```python
from build123d import *

# Parameters (mm, degrees)
BOSS_EXTRUDE1_DEPTH = 5
CUT_EXTRUDE1_DEPTH  = 44.153794735


with BuildPart() as part:
    # Sketch1 → Boss-Extrude1 (new body)
    with BuildSketch(Plane(origin=(0, 0, 0), x_dir=(1, 0, 0), z_dir=(0, 1, 0))):
        Polygon((-41, -5), (-41, 5), (-38, 5), (-38, 7.5), (-28.5, 7.5), (-28.5, 12.5), (-9.5, 12.5), (-9.5, 7.5), (0, 7.5), (0, -7.5), (-38, -7.5), (-38, -5), align=None)
    boss_extrude1 = extrude(amount=BOSS_EXTRUDE1_DEPTH)

    # Mirror1: Boss-Extrude1 across plane
    add(boss_extrude1.mirror(Plane(origin=(0, 5, -7.5), x_dir=(0, 0, 1), z_dir=(-1, 0, 0))))

    # Sketch4 → Cut-Extrude1 (cut, through all)
    with BuildSketch(Plane(origin=(0, 5, 0), x_dir=(1, 0, 0), z_dir=(0, 1, 0))):
        with BuildLine():
            Line((-33, -7.5), (33, -7.5))
            ThreePointArc((33, -7.5), (0, -2.5), (-33, -7.5))
        make_face()
    extrude(amount=-CUT_EXTRUDE1_DEPTH, mode=Mode.SUBTRACT)


solid = part.part
```
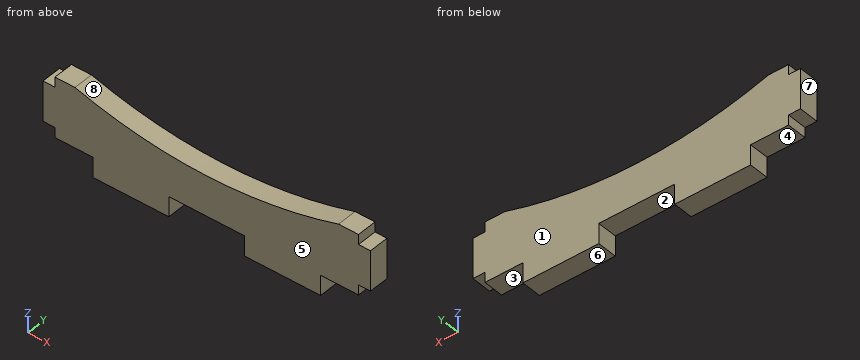
Geometry: final body of the model. Coordinates: model frame, mm. Face numbers are marked on the shaded views. A direction names the side the tool comes from. Give positions to 0.01 mm unless a question says otherwise; leave off trailing zeros. Loops run counter-clockwise (first coordinate to the right, second up) from the corner with the lowest first, then second, coordinate; pieces in that order, holes last. Notation, with made-up numbers: (38, 51.25) -> (75, 51.25) arc R14 ccw to (75, 59.25) -> close; hole circle Ø4 at (81.25, 54). An arc over 180 degrees is marked (long way). Return JSON: item names as keys, results as strings.
Item 1: Access query for the marked faces 1, 2, 3, 4 and 5. Directions: +Z, -Z, +X, -X, +Y, -Y. A direction counts if a zero-diameter tool reaches every point of the face in a straight line with its end or side. Return the directions, or none.
Filled in:
{"face 1": "+Z, -Z, +X, -X, +Y", "face 2": "-Z, +Y, -Y", "face 3": "-Z, +X, +Y, -Y", "face 4": "-Z, -X, +Y, -Y", "face 5": "+Z, -Z, +X, -X, -Y"}
Item 2: Mould query, pull axis X, two halves, no side actions, for the marked faces 6, 7 and 8. Classes: released by +X, released by -X, zero draft, split by the parting line, or undercut.
Filled in:
{"face 6": "zero draft", "face 7": "released by -X", "face 8": "undercut"}
Item 3: Section A-A, the plane y = 0.95. Output: boundary loops of the cut face in (x, z).
Filled in:
{"outline": "(-41, -5) -> (-38, -5) -> (-38, -7.5) -> (-28.5, -7.5) -> (-28.5, -12.5) -> (-9.5, -12.5) -> (-9.5, -7.5) -> (9.5, -7.5) -> (9.5, -12.5) -> (28.5, -12.5) -> (28.5, -7.5) -> (38, -7.5) -> (38, -5) -> (41, -5) -> (41, 5) -> (38, 5) -> (38, 7.5) -> (33, 7.5) arc R111.4 cw to (-33, 7.5) -> (-38, 7.5) -> (-38, 5) -> (-41, 5) -> close"}
Item 4: Section B-B, the plane x = 35.5. Output: boundary loops of the cut face in (y, z).
Filled in:
{"outline": "(0, -7.5) -> (5, -7.5) -> (5, 7.5) -> (0, 7.5) -> close"}
Item 5: Section C-C, the plane x = -12. Output: boundary loops of the cut face in (y, z), plus the area to 3 significant figures.
Filled in:
{"outline": "(0, -12.5) -> (5, -12.5) -> (5, 3.15) -> (0, 3.15) -> close", "area": "78.2 mm^2"}
Item 6: Line query: line 1 (X direction, y = 3.1, z = -7.75); line 2 (Z direction, x = 23.5, y = 2.75); line 3 (Z direction, x = -33, y = 3.75). Output: solid intervals per line, ascending.
Filled in:
{"line 1": "-28.5 to -9.5, 9.5 to 28.5", "line 2": "-12.5 to 5.01", "line 3": "-7.5 to 7.5"}
Item 7: Pin query (flat end, axial travel): P1, Ø12, axis at x = 6, z = -5.5, coming from the -Y side; P2, Ø1.5, axis at y = 3.5, z = -9, coming from the +X side; P3, Ø1.2, axis at y = 3, z = -6, coming from the -X side; P4, Ø1.5, axis at x = -39, y = 2, coming from the +Z side. Return the tip coordinate at first contact, or that it passes through.
Filled in:
{"P1": "y = 0", "P2": "x = 28.5", "P3": "x = -38", "P4": "z = 5"}
